Can you work these out from the model? Positions are in its coordinate system, mm. Give positions to 0.01 mm unless a question says otherwise; leave off trailing zeros. Order: outer loops, then holes, each group sorted by start corner. A loop starts at its lowest first (then second) coordinate and runs counter-clockwise, first axis right, second up. Notation, with made-up numbers: M 18.5,62.5 L 26.5,62.5 A24 cw 26.5,99.5 Z; hole C 44,65 d8. An arc over 180 degrees is marked long. Answer as a JSON object with one key per item and string values.
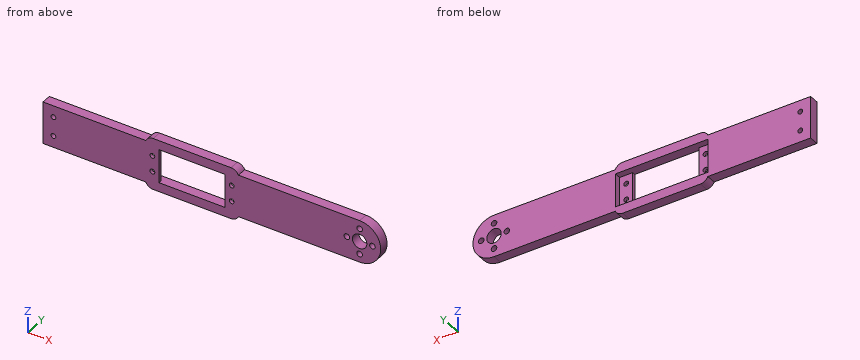
```python
from build123d import *

# Parameters (mm, degrees)
SKETCH1_W            = 57.629592668
SKETCH1_H            = 21.211867522
SKETCH1_R            = 1.75
SKETCH1_R_2          = 4.5
BOSS_EXTRUDE1_DEPTH  = 6
SKETCH1_22_W         = 8.129592668
SKETCH1_22_H         = 21.211867522
SKETCH1_22_R         = 1.5
BOSS_EXTRUDE2_DEPTH  = 2
SKETCH4_W            = 57.748953374
SKETCH4_H            = 6
BOSS_EXTRUDE4_DEPTH  = 3
FILLET2_R            = 5
FILLET2_OF_MIRROR1_R = 5
SKETCH8_R            = 1.5
CUT_EXTRUDE4_DEPTH   = 13


with BuildPart() as part:
    # Sketch1 → Boss-Extrude1 (new body)
    with BuildSketch(Plane(origin=(0, 0, 0), x_dir=(1, 0, 0), z_dir=(0, 1, 0))):
        with BuildLine():
            Line((-197.556308439, -13.154372872), (0, -13.154372872))
            ThreePointArc((0, -13.154372872), (13.154372872, 0), (0, 13.154372872))
            Line((0, 13.154372872), (-197.556308439, 13.154372872))
            Line((-197.556308439, 13.154372872), (-197.556308439, -13.154372872))
        make_face()
        with Locations((-104.57172107, -0.139435446)):
            Rectangle(SKETCH1_W, SKETCH1_H, mode=Mode.SUBTRACT)
        with Locations(Location((0, 8, 0), (0, 0, 270))):
            Circle(SKETCH1_R, mode=Mode.SUBTRACT)
        with Locations(Location((0, -8, 0), (0, 0, 270))):
            Circle(SKETCH1_R, mode=Mode.SUBTRACT)
        with Locations(Location((-8, 0, 0), (0, 0, 270))):
            Circle(SKETCH1_R, mode=Mode.SUBTRACT)
        with Locations(Location((0, 0, 0), (0, 0, 270))):
            Circle(SKETCH1_R_2, mode=Mode.SUBTRACT)
        with Locations(Location((8, 0, 0), (0, 0, 270))):
            Circle(SKETCH1_R, mode=Mode.SUBTRACT)
    boss_extrude1 = extrude(amount=BOSS_EXTRUDE1_DEPTH)

    # Sketch1<22> → Boss-Extrude2 (add)
    # profile 1 of 2: a face of its own
    with BuildSketch(Plane(origin=(0, 0, 0), x_dir=(1, 0, 0), z_dir=(0, 1, 0))):
        with Locations((-129.32172107, -0.139435446)):
            Rectangle(SKETCH1_22_W, SKETCH1_22_H)
        with Locations(Location((-129.32172107, -5, 0), (0, 0, 270))):
            Circle(SKETCH1_22_R, mode=Mode.SUBTRACT)
        with Locations(Location((-129.29672107, 5, 0), (0, 0, 270))):
            Circle(SKETCH1_22_R, mode=Mode.SUBTRACT)
    # profile 2 of 2: a face of its own
    with BuildSketch(Plane(origin=(0, 0, 0), x_dir=(1, 0, 0), z_dir=(0, 1, 0))):
        with Locations((-79.82172107, -0.139435446)):
            Rectangle(SKETCH1_22_W, SKETCH1_22_H)
        with Locations(Location((-79.82172107, -5, 0), (0, 0, 270))):
            Circle(SKETCH1_22_R, mode=Mode.SUBTRACT)
        with Locations(Location((-79.84672107, 5, 0), (0, 0, 270))):
            Circle(SKETCH1_22_R, mode=Mode.SUBTRACT)
    extrude(amount=BOSS_EXTRUDE2_DEPTH)

    # Sketch4 → Boss-Extrude4 (add)
    with BuildSketch(Plane.XY.offset(13.154372872)):
        with Locations((-104.509525291, 3)):
            Rectangle(SKETCH4_W, SKETCH4_H)
    boss_extrude4 = extrude(amount=BOSS_EXTRUDE4_DEPTH)

    # Fillet2
    # the kernel refuses this fillet: 5 mm, written as the material it takes off along each edge
    with BuildSketch(Plane(origin=(-75.635048604, -11.456439237, 16.154372872), x_dir=(0, 0, -1), z_dir=(0, 1, 0)), Plane(origin=(-133.384001978, 17.456439237, 16.154372872), x_dir=(0, 0, -1), z_dir=(0, -1, 0))) as fillet2_piece_1:
        with BuildLine():
            CenterArc((5, 4.582575695), FILLET2_R, 180, 66.421821522)
            Line((0, 4.582575695), (-0.1, 4.582575695))
            Line((-0.1, 4.582575695), (-0.1, 0))
            Line((-0.1, 0), (0, -0.1))
            ThreePointArc((0, -0.1), (1.5, -0.1), (2.96, -0.091651514))
            Line((2.96, -0.091651514), (3, 0))
        make_face()
    extrude(amount=28.912878475, mode=Mode.SUBTRACT)

    # Mirror1: Boss-Extrude1, Boss-Extrude4 across plane
    add(boss_extrude1.mirror(Plane(origin=(0, 0, 0), x_dir=(1, 0, 0), z_dir=(0, 0, -1))))
    add(boss_extrude4.mirror(Plane(origin=(0, 0, 0), x_dir=(1, 0, 0), z_dir=(0, 0, -1))))

    # Fillet2 of Mirror1
    # the kernel refuses this fillet: 5 mm, written as the material it takes off along each edge
    with BuildSketch(Plane(origin=(-75.635048604, -11.456439237, -16.154372872), x_dir=(0, 0, 1), z_dir=(0, 1, 0))) as fillet2_of_mirror1_piece_1:
        with BuildLine():
            CenterArc((5, -4.582575695), FILLET2_OF_MIRROR1_R, 113.578178478, 66.421821522)
            Line((0, -4.582575695), (-0.1, -4.582575695))
            Line((-0.1, -4.582575695), (-0.1, 0))
            Line((-0.1, 0), (0, 0.1))
            ThreePointArc((0, 0.1), (1.5, 0.1), (2.96, 0.091651514))
            Line((2.96, 0.091651514), (3, 0))
        make_face()
    extrude(amount=28.912878475, mode=Mode.SUBTRACT)
    with BuildSketch(Plane(origin=(-133.384001978, 17.456439237, -16.154372872), x_dir=(1, 0, 0), z_dir=(0, -1, 0))) as fillet2_of_mirror1_piece_2:
        with BuildLine():
            CenterArc((4.582575695, 5), FILLET2_OF_MIRROR1_R, 203.578178478, 66.421821522)
            Line((0, 3), (-0.091651514, 2.96))
            ThreePointArc((-0.091651514, 2.96), (-0.1, 1.5), (-0.1, 0))
            Line((-0.1, 0), (0, -0.1))
            Line((0, -0.1), (4.582575695, -0.1))
            Line((4.582575695, -0.1), (4.582575695, 0))
        make_face()
    extrude(amount=28.912878475, mode=Mode.SUBTRACT)

    # Sketch8 → Cut-Extrude4 (cut)
    with BuildSketch(Plane(origin=(0, 6, 0), x_dir=(1, 0, 0), z_dir=(0, 1, 0))):
        with Locations(Location((-191.056308439, -5.984372872, 0), (0, 0, 270))):
            Circle(SKETCH8_R)
        with Locations(Location((-191.056308439, 5.984372872, 0), (0, 0, 270))):
            Circle(SKETCH8_R)
    extrude(amount=-CUT_EXTRUDE4_DEPTH, mode=Mode.SUBTRACT)


solid = part.part
```
1) I want a section at D-D on x = 8. Write out the boundary of the cut face in (y, z).
Results found:
{"outline": "M 0,-10.44 L 6,-10.44 L 6,-1.75 L 0,-1.75 Z; M 0,1.75 L 6,1.75 L 6,10.44 L 0,10.44 Z"}
2) I need wall thicknesses on L1, parallel to X at y = 3.8, z = 0; L2, parallel to Z at x = -99.5, y = 3; L3, parallel to X at y = 2.35, z = -1. Which ranges of each line are inside material? Lowest first, please.
Results found:
{"L1": "x = -197.56 to -133.39, -75.76 to -9.75, -6.25 to -4.5, 4.5 to 6.25, 9.75 to 13.15", "L2": "z = -16.15 to -10.47, 10.47 to 16.15", "L3": "x = -197.56 to -133.39, -75.76 to -9.44, -6.56 to -4.39, 4.39 to 6.56, 9.44 to 13.12"}
3) I'm going to push flat-ended pins straight in: pin 1 Ø1.6 at (y, z) = (1, 4) entering from +X; pin 2 Ø1.2 at (y, z) = (4.5, -4) entering from +X; pin 3 Ø11.5 at (x, z) = (0, 0) entering from +Y; pin 4 Ø4 at (x, z) = (-129.3, -5) entering from +Y. Where does each tip first touch, or does it pass through?
Results found:
{"pin 1": "stops at x = 12.76", "pin 2": "stops at x = 12.71", "pin 3": "stops at y = 6", "pin 4": "stops at y = 2"}
4) I want a section at B-B on x = -117. Write out the boundary of the cut face in (y, z), and give its area (3 significant figures).
Results found:
{"outline": "M 0,-16.15 L 6,-16.15 L 6,-10.47 L 0,-10.47 Z; M 0,10.47 L 6,10.47 L 6,16.15 L 0,16.15 Z", "area": "68.3 mm²"}
5) I want a section at A-A on z = 0. Write out the boundary of the cut face in (x, y), and give its area (3 significant figures).
Results found:
{"outline": "M -197.56,0 L -125.26,0 L -125.26,2 L -133.39,2 L -133.39,6 L -197.56,6 Z; M -83.89,0 L -9.75,0 L -9.75,6 L -75.76,6 L -75.76,2 L -83.89,2 Z; M -6.25,0 L -4.5,0 L -4.5,6 L -6.25,6 Z; M 4.5,0 L 6.25,0 L 6.25,6 L 4.5,6 Z; M 9.75,0 L 13.15,0 L 13.15,6 L 9.75,6 Z", "area": "855 mm²"}
6) I want a section at C-C on y = 1. Count the separate pieces of the cut face and the enclosed holes in it, and give its area (3 significant figures).
Results found:
{"separate pieces": "1", "enclosed holes": "12", "area": "4,790 mm²"}
